CAD build for the part. Positions are in the model's coordinates, mm. Give positions to 0.01 mm unless a question says otherwise; leave off trailing zeros. Order: outer loops, then holes, each group sorted by start corner. A loop starts at its lowest first (then second) coordinate and runs counter-clockwise, first axis right, second up. Notation, with made-up numbers: (20.5, 59.25) -> (32.5, 59.25) arc R34 ccw to (32.5, 89.25) -> close; hole circle Ø6 at (16, -4). An arc over 180 degrees is marked (long way). Use one line per item in the form item = value. Start each with the question number.
1) Probe line 1 (Y direction, x = 0.1, z = -20); line 2 (Z direction, x = -0.6, y = 1.45); line 3 (X direction, y = -1.55, z = 11). List the from-to ranges inside material, lowest first.
2) Cut at A-A, the plane z = -14.5. Give the cut face in (x, y), and give its area (3 significant figures).
3) Drop flat-ended pins along their axis: P1, Ø1.5, axis at y = -1, z = -12, coming from the +X side; P2, Ø1, axis at y = -1, z = 8.5, coming from the -X side. Give the stop position or say it passes through.
Autodesk Inventor part; units mm, degrees
sketch "スケッチ1" plane through (0, 0, 0) normal (0, 0, 1) x (1, 0, 0)
  circle A0 centre (0, 0) radius 2
  dimension "d0" = 4
extrude "押し出し1" add sketch "スケッチ1" along normal mid plane 45
chamfer "面取り1" distance 0.5 angle 45 1 edges at (-2, 0, 22.5)
chamfer "面取り2" distance 0.5 angle 45 1 edges at (-2, 0, -22.5)
properties part number "shaft4x45"
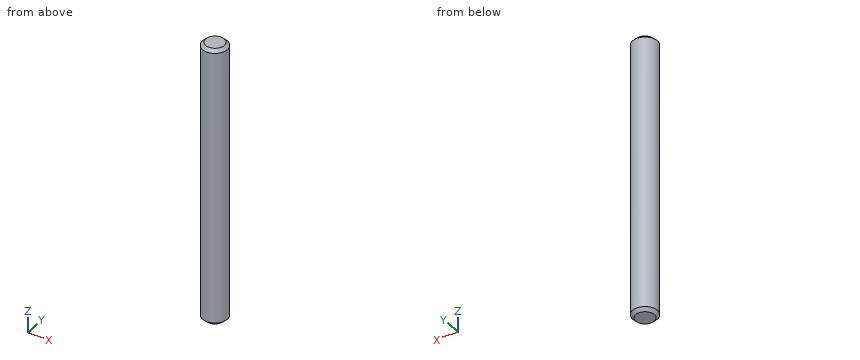
Result:
q1.line_1 = -2 to 2
q1.line_2 = -22.43 to 22.43
q1.line_3 = -1.26 to 1.26
q2.outline = circle Ø4 at (0, 0)
q2.area = 12.6 mm²
q3.P1 = 1.98
q3.P2 = -1.94
